```python
from build123d import *

# Parameters (mm, degrees)
BOSS_EXTRUDE1_DEPTH = 50
CUT_EXTRUDE1_REACH  = 5
SKETCH2_R           = 11.05
SKETCH2_R_2         = 1.75
CUT_EXTRUDE2_REACH  = 5
CHAMFER1_SIZE       = 5


with BuildPart() as part:
    # Sketch1 → Boss-Extrude1 (new body)
    with BuildSketch(Plane(origin=(0, 0, 0), x_dir=(0, 0, -1), z_dir=(1, 0, 0))):
        Polygon((0, 0), (0, 3), (50, 3), (50, 51), (53, 51), (53, 0), align=None)
    extrude(amount=-BOSS_EXTRUDE1_DEPTH)

    # Sketch2 → Cut-Extrude1 (cut, up to next)
    with BuildSketch(Plane.XY.offset(-50), mode=Mode.PRIVATE) as cut_extrude1_sk1:
        with Locations((-25, 27)):
            Circle(SKETCH2_R)
    cut_extrude1_tool1 = extrude(cut_extrude1_sk1.sketch, amount=-CUT_EXTRUDE1_REACH, mode=Mode.PRIVATE) & part.part
    add(cut_extrude1_tool1.solids().sort_by_distance((-25, 27, -50))[0], mode=Mode.SUBTRACT)
    # Sketch2 → Cut-Extrude1 (cut, up to next)
    with BuildSketch(Plane.XY.offset(-50), mode=Mode.PRIVATE) as cut_extrude1_sk2:
        with Locations((-40.5, 42.5)):
            Circle(SKETCH2_R_2)
    cut_extrude1_tool2 = extrude(cut_extrude1_sk2.sketch, amount=-CUT_EXTRUDE1_REACH, mode=Mode.PRIVATE) & part.part
    add(cut_extrude1_tool2.solids().sort_by_distance((-40.5, 42.5, -50))[0], mode=Mode.SUBTRACT)
    # Sketch2 → Cut-Extrude1 (cut, up to next)
    with BuildSketch(Plane.XY.offset(-50), mode=Mode.PRIVATE) as cut_extrude1_sk3:
        with Locations((-9.5, 42.5)):
            Circle(SKETCH2_R_2)
    cut_extrude1_tool3 = extrude(cut_extrude1_sk3.sketch, amount=-CUT_EXTRUDE1_REACH, mode=Mode.PRIVATE) & part.part
    add(cut_extrude1_tool3.solids().sort_by_distance((-9.5, 42.5, -50))[0], mode=Mode.SUBTRACT)
    # Sketch2 → Cut-Extrude1 (cut, up to next)
    with BuildSketch(Plane.XY.offset(-50), mode=Mode.PRIVATE) as cut_extrude1_sk4:
        with Locations((-9.5, 11.5)):
            Circle(SKETCH2_R_2)
    cut_extrude1_tool4 = extrude(cut_extrude1_sk4.sketch, amount=-CUT_EXTRUDE1_REACH, mode=Mode.PRIVATE) & part.part
    add(cut_extrude1_tool4.solids().sort_by_distance((-9.5, 11.5, -50))[0], mode=Mode.SUBTRACT)
    # Sketch2 → Cut-Extrude1 (cut, up to next)
    with BuildSketch(Plane.XY.offset(-50), mode=Mode.PRIVATE) as cut_extrude1_sk5:
        with Locations((-40.5, 11.5)):
            Circle(SKETCH2_R_2)
    cut_extrude1_tool5 = extrude(cut_extrude1_sk5.sketch, amount=-CUT_EXTRUDE1_REACH, mode=Mode.PRIVATE) & part.part
    add(cut_extrude1_tool5.solids().sort_by_distance((-40.5, 11.5, -50))[0], mode=Mode.SUBTRACT)

    # Sketch3 → Cut-Extrude2 (cut, up to next)
    with BuildSketch(Plane(origin=(0, 3, 0), x_dir=(1, 0, 0), z_dir=(0, 1, 0)), mode=Mode.PRIVATE) as cut_extrude2_sk1:
        with BuildLine():
            Line((-37.9, 40), (-37.9, 10))
            ThreePointArc((-37.9, 10), (-40, 7.9), (-42.1, 10))
            Line((-42.1, 10), (-42.1, 40))
            ThreePointArc((-42.1, 40), (-40, 42.1), (-37.9, 40))
        make_face()
    cut_extrude2_tool1 = extrude(cut_extrude2_sk1.sketch, amount=-CUT_EXTRUDE2_REACH, mode=Mode.PRIVATE) & part.part
    add(cut_extrude2_tool1.solids().sort_by_distance((-40, 3, -25))[0], mode=Mode.SUBTRACT)
    # Sketch3 → Cut-Extrude2 (cut, up to next)
    with BuildSketch(Plane(origin=(0, 3, 0), x_dir=(1, 0, 0), z_dir=(0, 1, 0)), mode=Mode.PRIVATE) as cut_extrude2_sk2:
        with BuildLine():
            Line((-12.1, 40), (-12.1, 10))
            ThreePointArc((-12.1, 10), (-10, 7.9), (-7.9, 10))
            Line((-7.9, 10), (-7.9, 40))
            ThreePointArc((-7.9, 40), (-10, 42.1), (-12.1, 40))
        make_face()
    cut_extrude2_tool2 = extrude(cut_extrude2_sk2.sketch, amount=-CUT_EXTRUDE2_REACH, mode=Mode.PRIVATE) & part.part
    add(cut_extrude2_tool2.solids().sort_by_distance((-10, 3, -25))[0], mode=Mode.SUBTRACT)

    # Chamfer1
    chamfer1_edges = [part.edges().sort_by_distance(p)[0] for p in [
        (-50, 51, -51.5),
        (-50, 1.5, 0),
        (0, 1.5, 0),
        (0, 51, -51.5),
    ]]
    chamfer(chamfer1_edges, length=CHAMFER1_SIZE)


solid = part.part
```
Verification items for the finished model (mm, model axes). A direction names the side the tool comes from. Round coordinates to 2 decimals unless told otherwise and drop trailing zeros. Order: outer loops, then holes, each group sorted by start corner. A loop starts at its lowest first (then second) coordinate and runs counter-clockwise, first axis right, second up. Notation, with made-up numbers: (78.25, -27.5) -> (116.25, -27.5) arc R5 cw to (116.25, -20.5) -> close; hole circle Ø10 at (41.25, -19.75). An arc over 180 degrees is marked (long way). Put each result on its own line as item: value. Start each with the question number.
(1) Draft check along X on faces 4 (the face through (-14.79, 22.77, -51.48)), 5 (the face through (-47, 49, -51)), 6 (the face through (-25, 3, -25)). Enter one of: +X half, -X half, draft (parallel to the pull), parting line (faces both ways), or undercut.
(2) Section check A-A (y = 11.5). Enter the section's corners in (x, z), then the cut area to 3 significant figures.
(3) Material ranges on line 1 along Y through (x, z) = (-40.5, -50.8); line 2 along Y through (x, z) = (-26, -9); line 3 along X through (y, z) = (42, -52), recorded low to high.
(4) Section check C-C (x = -25). Enter the section's corners in (y, z), then the cut area to 3 significant figures.
(5) Tool access check on faces 1 (the face through (-40, 1.5, -42.1)), 2 (the face through (-13.5, 26.7, -50)), 3 (the face through (-25, 0, -27)). Record the directions out of +Z, -Z, +X, -X, +Y, -Y that give a thin tool (end or side, any length) a straight path to the whole face; none if there is none.
(6) Section check D-D (y = 27). Enter the section's corners in (x, z).
(7) Depth check by flat-ended pin: pin 1 Ø4.5 at (x, y) = (-40.5, 11.5) entering from +Z; pin 2 Ø2 at (x, z) = (-18.5, -29) entering from +Y. Enter the tip coordinate at first touch or a pass-through.
(8) Section check B-B (z = -11). Enter the section's corners in (x, y).
Completed:
1. face 4: undercut
1. face 5: -X half
1. face 6: draft
2. outline: (-50, -53) -> (-42.25, -53) -> (-42.25, -50) -> (-50, -50) -> close; (-38.75, -53) -> (-11.25, -53) -> (-11.25, -50) -> (-38.75, -50) -> close; (-7.75, -53) -> (0, -53) -> (0, -50) -> (-7.75, -50) -> close
2. area: 129 mm2
3. line 1: y = 0 to 9.75, 13.25 to 40.75, 44.25 to 51
3. line 2: y = 0 to 3
3. line 3: x = -50 to -42.18, -38.82 to -11.18, -7.82 to 0
4. outline: (0, -53) -> (15.95, -53) -> (15.95, -50) -> (3, -50) -> (3, 0) -> (0, 0) -> close; (38.05, -53) -> (51, -53) -> (51, -50) -> (38.05, -50) -> close
4. area: 237 mm2
5. face 1: +Y, -Y
5. face 2: +Z, +X, -X, +Y
5. face 3: +Z, -Z, +X, -X, -Y
6. outline: (-50, -53) -> (-36.05, -53) -> (-36.05, -50) -> (-50, -50) -> close; (-13.95, -53) -> (0, -53) -> (0, -50) -> (-13.95, -50) -> close
7. pin 1: stops at z = -50
7. pin 2: stops at y = 3
8. outline: (-50, 0) -> (-42.1, 0) -> (-42.1, 3) -> (-50, 3) -> close; (-37.9, 0) -> (-12.1, 0) -> (-12.1, 3) -> (-37.9, 3) -> close; (-7.9, 0) -> (0, 0) -> (0, 3) -> (-7.9, 3) -> close
